Here's how the part is built. I have some questions about the finished solid (model axes, mm). A direction names the side the tool comes from. Give positions to 0.01 mm unless a question says otherwise; leave off trailing zeros. Loops run counter-clockwise (first coordinate to the right, second up) from the corner with the lowest first, then second, coordinate; pieces in that order, holes last.
Q1. I'm going to push flat-ended pins straight in: P1, Ø2.5, axis at x = 245, y = 345, coming from the +Z side; P2, Ø14.5, axis at x = 236.5, y = 12, coming from the +Z side; P3, Ø1.5, axis at x = 107, z = 22, coming from the -Y side. Where does each tip first touch, or does it pass through?
Q2. Thinking about a two-plate mould opening in Z: for faces 1 (the face through (7, 11, 11)), 2 (the face through (228.373, 352.961, 14.65)), 3 (the face through (231.277, 14.302, 5.423)), which applies, pulls with the +Z half, pulls with the -Z half, needs draft (parallel to the pull), parting line crosses it, or undercut?
Q3. Suppose I cut it at B-B (y = 195). List the corners of the cut face in (x, z) for me.
Q4. I need wall thicknesses on probe 1 along X at (y, z) = (110, 12.25); probe 2 along X at (y, z) = (66.5, 16.75); probe 3 along X at (y, z) = (299.5, 8). Which ranges of each line are inside material? Lowest first, please.
Q5. For faces 4 (the face through (235.1, 6.6, 11)), 5 (the face through (191.5, 193, 5)), 6 (the face through (65, 193, 18)), 7 (the face through (91.095, 352.961, 11.633)), which set-ups out of +Z, -Z, +X, -X, +Y, -Y let a thin tool reach every point of the face, with its end or its side?
Q6. Suppose I cut it at A-A (y = 12.5). Count the separate pieces of the cut face and the enclosed holes in it, and give its area (3 significant figures).
```python
from build123d import *

# Parameters (mm, degrees)
SKETCH_1_W          = 250
SKETCH_1_H          = 380
SKETCH_1_R          = 9
SKETCH_1_R_2        = 2
SKETCH_1_R_3        = 1.5
SKETCH_1_R_4        = 3
EXTRUDE_3_DEPTH     = 25
CUT_EXTRUDE_1_DEPTH = 416
SKETCH_3_4_R        = 4
CUT_EXTRUDE_2_DEPTH = 55
SKETCH_5_W          = 76.418543054
SKETCH_5_H          = 18.162254628
EXTRUDE_4_DEPTH     = 12
SKETCH_6_W          = 9.937837438
SKETCH_6_H          = 197.728696601
EXTRUDE_5_DEPTH     = 12
SKETCH_7_W          = 21.060874429
SKETCH_7_H          = 111.734651623
EXTRUDE_6_DEPTH     = 12
SKETCH_8_W          = 15.76346628
SKETCH_8_H          = 76.418543054
EXTRUDE_7_DEPTH     = 5
SKETCH_9_W          = 10.965889587
SKETCH_9_H          = 75.390490905
EXTRUDE_8_DEPTH     = 5
SKETCH_10_W         = 21.30480461
SKETCH_10_H         = 26.996927979
SKETCH_10_R         = 6
EXTRUDE_11_DEPTH    = 11
FILLET_1_R          = 4
SKETCH_11_R         = 2
CUT_EXTRUDE_3_DEPTH = 13


with BuildPart() as part:
    # 草图1 → 凸台-拉伸3 (new body)
    with BuildSketch(Plane.XY):
        with Locations((125.613842041, 190.076299127)):
            Rectangle(SKETCH_1_W, SKETCH_1_H)
        with Locations((13, 12.5)):
            Circle(SKETCH_1_R, mode=Mode.SUBTRACT)
        with Locations((237, 12.5)):
            Circle(SKETCH_1_R, mode=Mode.SUBTRACT)
        with Locations((5, 360)):
            Circle(SKETCH_1_R_2, mode=Mode.SUBTRACT)
        with Locations((5, 260)):
            Circle(SKETCH_1_R_2, mode=Mode.SUBTRACT)
        with Locations((15, 360)):
            Circle(SKETCH_1_R_2, mode=Mode.SUBTRACT)
        with Locations((15, 260)):
            Circle(SKETCH_1_R_2, mode=Mode.SUBTRACT)
        with Locations((89, 280)):
            Circle(SKETCH_1_R_3, mode=Mode.SUBTRACT)
        with Locations((113, 280)):
            Circle(SKETCH_1_R_3, mode=Mode.SUBTRACT)
        with Locations((137, 280)):
            Circle(SKETCH_1_R_3, mode=Mode.SUBTRACT)
        with Locations((161, 280)):
            Circle(SKETCH_1_R_3, mode=Mode.SUBTRACT)
        with Locations((45, 110)):
            Circle(SKETCH_1_R_4, mode=Mode.SUBTRACT)
        with Locations((45, 170)):
            Circle(SKETCH_1_R_4, mode=Mode.SUBTRACT)
        with Locations((205, 170)):
            Circle(SKETCH_1_R_4, mode=Mode.SUBTRACT)
        with Locations((205, 110)):
            Circle(SKETCH_1_R_4, mode=Mode.SUBTRACT)
        with Locations((245, 345)):
            Circle(SKETCH_1_R_3, mode=Mode.SUBTRACT)
        with Locations((245, 285)):
            Circle(SKETCH_1_R_3, mode=Mode.SUBTRACT)
        with Locations((245, 225)):
            Circle(SKETCH_1_R_3, mode=Mode.SUBTRACT)
        with Locations((245, 165)):
            Circle(SKETCH_1_R_3, mode=Mode.SUBTRACT)
    extrude(amount=EXTRUDE_3_DEPTH)

    # 草图3 → 切除-拉伸1 (cut)
    with BuildSketch(Plane(origin=(0, 380.076299127, 0), x_dir=(1, 0, 0), z_dir=(0, 1, 0))):
        Polygon((71.5, -9), (71.5, 0), (58.5, 0), (58.5, -9), (55, -9), (55, -18), (75, -18), (75, -9), align=None)
        Polygon((191.5, 0), (178.5, 0), (178.5, -9), (175, -9), (175, -18), (195, -18), (195, -9), (191.5, -9), align=None)
    extrude(amount=-CUT_EXTRUDE_1_DEPTH, mode=Mode.SUBTRACT)

    # 草图3<4> → 切除-拉伸2 (cut)
    with BuildSketch(Plane(origin=(0, 380.076299127, 0), x_dir=(1, 0, 0), z_dir=(0, 1, 0))):
        with Locations(Location((95, -12.5, 0), (0, 0, 270))):
            Circle(SKETCH_3_4_R)
        with Locations(Location((155, -12.5, 0), (0, 0, 270))):
            Circle(SKETCH_3_4_R)
        with Locations(Location((225, -12.5, 0), (0, 0, 270))):
            Circle(SKETCH_3_4_R)
        with Locations(Location((25, -12.5, 0), (0, 0, 270))):
            Circle(SKETCH_3_4_R)
    extrude(amount=-CUT_EXTRUDE_2_DEPTH, mode=Mode.SUBTRACT)

    # 草图5 → 凸台-拉伸4 (add)
    with BuildSketch(Plane(origin=(0, 0, 0), x_dir=(-1, 0, 0), z_dir=(0, 0, -1))):
        with Locations((-124.414447867, 279.859520114)):
            Rectangle(SKETCH_5_W, SKETCH_5_H)
    extrude(amount=-EXTRUDE_4_DEPTH)

    # 草图6 → 凸台-拉伸5 (add)
    with BuildSketch(Plane(origin=(0, 0, 0), x_dir=(-1, 0, 0), z_dir=(0, 0, -1))):
        with Locations((-244.34867248, 253.130164248)):
            Rectangle(SKETCH_6_W, SKETCH_6_H)
    extrude(amount=-EXTRUDE_5_DEPTH)

    # 草图7 → 凸台-拉伸6 (add)
    with BuildSketch(Plane(origin=(0, 0, 0), x_dir=(-1, 0, 0), z_dir=(0, 0, -1))):
        with Locations((-11.144279256, 310.45109449)):
            Rectangle(SKETCH_7_W, SKETCH_7_H)
    extrude(amount=-EXTRUDE_6_DEPTH)

    # 草图8 → 凸台-拉伸7 (add)
    with BuildSketch(Plane(origin=(0, 0, 0), x_dir=(-1, 0, 0), z_dir=(0, 0, -1))):
        with Locations((-204.431173441, 138.673691692)):
            Rectangle(SKETCH_8_W, SKETCH_8_H)
    extrude(amount=-EXTRUDE_7_DEPTH)

    # 草图9 → 凸台-拉伸8 (add)
    with BuildSketch(Plane(origin=(0, 0, 0), x_dir=(-1, 0, 0), z_dir=(0, 0, -1))):
        with Locations((-45.425774442, 139.530401815)):
            Rectangle(SKETCH_9_W, SKETCH_9_H)
    extrude(amount=-EXTRUDE_8_DEPTH)

    # 草图10 → 凸台-拉伸11 (add)
    # profile 1 of 2: a face of its own
    with BuildSketch(Plane(origin=(0, 0, 0), x_dir=(-1, 0, 0), z_dir=(0, 0, -1))):
        with Locations((-236.946967286, 15.123600302)):
            Rectangle(SKETCH_10_W, SKETCH_10_H)
        with Locations((-237, 12.5)):
            Circle(SKETCH_10_R, mode=Mode.SUBTRACT)
    # profile 2 of 2: a face of its own
    with BuildSketch(Plane(origin=(0, 0, 0), x_dir=(-1, 0, 0), z_dir=(0, 0, -1))):
        with Locations((-13.053032714, 15.123600302)):
            Rectangle(SKETCH_10_W, SKETCH_10_H)
        with Locations((-13, 12.5)):
            Circle(SKETCH_10_R, mode=Mode.SUBTRACT)
    extrude(amount=-EXTRUDE_11_DEPTH)

    # 圆角1
    # the kernel refuses this fillet: 4 mm, written as the material it takes off along each edge
    with BuildSketch(Plane(origin=(-9.386157959, 0.076299127, 25), x_dir=(0, 0, -1), z_dir=(1, 0, 0))) as fillet_1_piece_1:
        with BuildLine():
            CenterArc((FILLET_1_R, FILLET_1_R), FILLET_1_R, 180, 90)
            Line((0, FILLET_1_R), (0, 0))
            Line((0, 0), (FILLET_1_R, 0))
        make_face()
    extrude(amount=270, mode=Mode.SUBTRACT)

    # 草图11 → 切除-拉伸3 (cut)
    with BuildSketch(Plane.XY.offset(25)):
        with Locations((153.363842041, 160.076299127)):
            Circle(SKETCH_11_R)
        with Locations((97.863842041, 160.076299127)):
            Circle(SKETCH_11_R)
    extrude(amount=-CUT_EXTRUDE_3_DEPTH, mode=Mode.SUBTRACT)


solid = part.part
```
Solutions:
1. P1: stops at z = 12
1. P2: stops at z = 11
1. P3: stops at y = 0.08
2. face 1: pulls with the +Z half
2. face 2: undercut
2. face 3: needs draft
3. outline: (0.61, 0) - (58.5, 0) - (58.5, 9) - (55, 9) - (55, 18) - (75, 18) - (75, 9) - (71.5, 9) - (71.5, 0) - (178.5, 0) - (178.5, 9) - (175, 9) - (175, 18) - (195, 18) - (195, 9) - (191.5, 9) - (191.5, 0) - (250.61, 0) - (250.61, 25) - (0.61, 25) - close
4. probe 1: x = 0.61 to 42, 48 to 55, 75 to 175, 195 to 202, 208 to 250.61
4. probe 2: x = 0.61 to 55, 75 to 175, 195 to 250.61
4. probe 3: x = 0.61 to 58.5, 71.5 to 178.5, 191.5 to 250.61
5. face 4: +Z
5. face 5: -Z, +Y, -Y
5. face 6: +Y, -Y
5. face 7: +Y
6. separate pieces: 3
6. enclosed holes: 0
6. area: 4,890 mm2
